```python
from build123d import *

# Parameters (mm, degrees)
SKETCH1_W           = 31
SKETCH1_H           = 31
BOSS_EXTRUDE1_DEPTH = 1.5
SKETCH2_W           = 8
SKETCH2_H           = 8
BOSS_EXTRUDE2_DEPTH = 1.5
SKETCH3_R           = 4
BOSS_EXTRUDE3_DEPTH = 1.5
SKETCH4_W           = 7.4
SKETCH4_H           = 5.5
BOSS_EXTRUDE4_DEPTH = 3
SKETCH5_R           = 1.25
CUT_EXTRUDE1_DEPTH  = 23.12464689


with BuildPart() as part:
    # Sketch1 → Boss-Extrude1 (new body)
    with BuildSketch(Plane(origin=(0, 0, 0), x_dir=(1, 0, 0), z_dir=(0, 1, 0))):
        Rectangle(SKETCH1_W, SKETCH1_H)
    extrude(amount=BOSS_EXTRUDE1_DEPTH)

    # Sketch2 → Boss-Extrude2 (add)
    with BuildSketch(Plane(origin=(0, 1.5, 0), x_dir=(1, 0, 0), z_dir=(0, 1, 0))):
        Rectangle(SKETCH2_W, SKETCH2_H)
    extrude(amount=BOSS_EXTRUDE2_DEPTH)

    # Sketch3 → Boss-Extrude3 (add)
    with BuildSketch(Plane(origin=(0, 3, 0), x_dir=(1, 0, 0), z_dir=(0, 1, 0))):
        with Locations(Location((0, 0, 0), (0, 0, 270))):
            Circle(SKETCH3_R)
    extrude(amount=BOSS_EXTRUDE3_DEPTH)

    # Sketch4 → Boss-Extrude4 (add)
    with BuildSketch(Plane(origin=(0, 1.5, 0), x_dir=(1, 0, 0), z_dir=(0, 1, 0))):
        with Locations((0, -12.75)):
            Rectangle(SKETCH4_W, SKETCH4_H)
    extrude(amount=BOSS_EXTRUDE4_DEPTH)

    # Sketch5 → Cut-Extrude1 (cut, through all)
    with BuildSketch(Plane(origin=(0, 1.5, 0), x_dir=(1, 0, 0), z_dir=(0, 1, 0))):
        with Locations(Location((-14, 14, 0), (0, 0, 270))):
            Circle(SKETCH5_R)
        with Locations(Location((14, 14, 0), (0, 0, 270))):
            Circle(SKETCH5_R)
        with Locations(Location((14, -14, 0), (0, 0, 270))):
            Circle(SKETCH5_R)
        with Locations(Location((-14, -14, 0), (0, 0, 270))):
            Circle(SKETCH5_R)
    extrude(amount=-CUT_EXTRUDE1_DEPTH, mode=Mode.SUBTRACT)


solid = part.part
```
Check sheet for the modelled part. Datum: model origin and axes. Units: mm. A direction names the side the tool comes from. Give positions to 0.01 mm unless a question says otherwise; leave off trailing zeros. Order: outer loops, then holes, each group sorted by start corner. A loop starts at its lowest first (then second) coordinate and runs counter-clockwise, first axis right, second up. Notation, with made-up numbers: (65.25, 82) -> (115.25, 82) arc R13 cw to (115.25, 105) -> close; hole circle Ø6 at (67.5, 74.25). An arc over 180 degrees is marked (long way). Return JSON: item names as keys, results as strings.
1. Set-up check for faces 5 (the flat face through (0, 2, -4)), 6 (the flat face through (-3, 3, -3)), 7 (the flat face through (0, 3, 10)), 8 (the flat face through (-4, 2, 0)), 9 (the flat face through (3.7, 3, 13)): record each of +Z, -Z, +X, -X, +Y, -Y from which the full face is reachable in a straight line by a thin tool's end or side.
From the geometry:
{"face 5": "-Z, +X, -X, +Y", "face 6": "-Z, -X, +Y", "face 7": "+X, -X, +Y", "face 8": "+Z, -Z, -X, +Y", "face 9": "+Z, +X, +Y"}
2. Cross-section at C-C, the plane y = 4. Record the cut outline in (x, z).
From the geometry:
{"outline": "circle Ø8 at (0, 0); (-3.7, 10) -> (3.7, 10) -> (3.7, 15.5) -> (-3.7, 15.5) -> close"}
3. Cross-section at A-A, the plane z = -14. Record the cut outline in (x, y), plus the area to 3 significant figures.
From the geometry:
{"outline": "(-15.5, 0) -> (-15.25, 0) -> (-15.25, 1.5) -> (-15.5, 1.5) -> close; (-12.75, 0) -> (12.75, 0) -> (12.75, 1.5) -> (-12.75, 1.5) -> close; (15.25, 0) -> (15.5, 0) -> (15.5, 1.5) -> (15.25, 1.5) -> close", "area": "39.0 mm^2"}
4. Material ranges on probe 1 along X at (y, z) = (0.95, -14); probe 2 along Z at (x, y) = (13.5, 0.35); probe 3 along Y at (x, z) = (-11, 7), recorded low to high. Write a range as [from, to].
From the geometry:
{"probe 1": "[-15.5, -15.25], [-12.75, 12.75], [15.25, 15.5]", "probe 2": "[-15.5, -15.15], [-12.85, 12.85], [15.15, 15.5]", "probe 3": "[0, 1.5]"}
5. Cross-section at B-B, the plane x = 14. Record the cut outline in (y, z).
From the geometry:
{"outline": "(0, -15.5) -> (1.5, -15.5) -> (1.5, -15.25) -> (0, -15.25) -> close; (0, -12.75) -> (1.5, -12.75) -> (1.5, 12.75) -> (0, 12.75) -> close; (0, 15.25) -> (1.5, 15.25) -> (1.5, 15.5) -> (0, 15.5) -> close"}
6. Cross-section at D-D, the plane z = 14. Record the cut outline in (x, y), plus the area to 3 significant figures.
From the geometry:
{"outline": "(-15.5, 0) -> (-15.25, 0) -> (-15.25, 1.5) -> (-15.5, 1.5) -> close; (-12.75, 0) -> (12.75, 0) -> (12.75, 1.5) -> (3.7, 1.5) -> (3.7, 4.5) -> (-3.7, 4.5) -> (-3.7, 1.5) -> (-12.75, 1.5) -> close; (15.25, 0) -> (15.5, 0) -> (15.5, 1.5) -> (15.25, 1.5) -> close", "area": "61.2 mm^2"}
7. Mould release check, pull along X, two halves, no side actions. Record for faces 1 (the flat face through (-15.5, 1, 0)), 2 (the flat face through (15.5, 1, 0)), 3 (the cylindrical face through (15.24, 0.76, -14.16)), 4 (the cylindrical face through (15.24, 0.76, 13.84)): +X half, -X half, draft (parallel to the pull), parting line (faces both ways), or undercut.
From the geometry:
{"face 1": "-X half", "face 2": "+X half", "face 3": "undercut", "face 4": "undercut"}
8. Go/stop test with flat-tipped pins: P1, Ø5, axis at x = 4, z = -10.5, coming from the +Y side; P2, Ø0.8, axis at y = 2.5, z = -0.5, coming from the +X side; P3, Ø1.5, axis at y = 3.5, z = 11.5, coming from the -X side. Record where each tip stops, or that it passes through.
From the geometry:
{"P1": "y = 1.5", "P2": "x = 4", "P3": "x = -3.7"}
